CAD build for the part. Positions are in the model's coordinates, mm. Face numbers are marked on the shaded views. A direction names the side the tool comes from. Round coordinates to 2 decimals unless told otherwise and drop trailing zeros. Write each loop counter-clockwise with the first axis right and the second up, starting at its lowest first coordinate (ties: lowest second). Pieces come first, ordered by that corner, then holes. Notation, with made-up numbers: (30, 42) - (49, 42) arc R16 cw to (49, 66) - close; hole circle Ø9 at (69.5, -4.5). An arc over 180 degrees is marked (long way). Put each result on its own line as item: value. Start each with the question number.
Item 1: Mould opens along X. For the marked faces 4, 5 and 6 say: released by +X, released by -X, zero draft, split by the parting line, or undercut.
Item 2: Cut at B-B (x = 58). Give the cut face in (y, z), and give its area (3 significant figures).
Item 3: Pin check, flat tips, straight feed: pin 1 Ø2 at (x, z) = (11.5, 50.5) entering from -Y; pin 2 Ø12.5 at (y, z) = (-43, -43) entering from +X; pin 3 Ø5 at (y, z) = (51.5, 5.5) entering from +X; pin 4 Ø16 at (y, z) = (43, -43) entering from +X. Stop position of each tip, or through.
Item 4: Cut at A-A (z = 59.5). Give the cut face in (x, y).
Item 5: 3-axis set-ups, long thin cutter, end or side, ignore diameter. For the marked faces 1, 2 and 3: which of +Z, -Z, +X, -X, +Y, -Y reach the whole face in a straight line?
Item 6: Drill centre lines: line 1 (Y direction, x = 10.5, z = 43); line 2 (X direction, y = 36, z = -19); line 3 (Y direction, x = 58.5, z = 40). Where is each one in solid material? Low to high. Write a range as from..to.
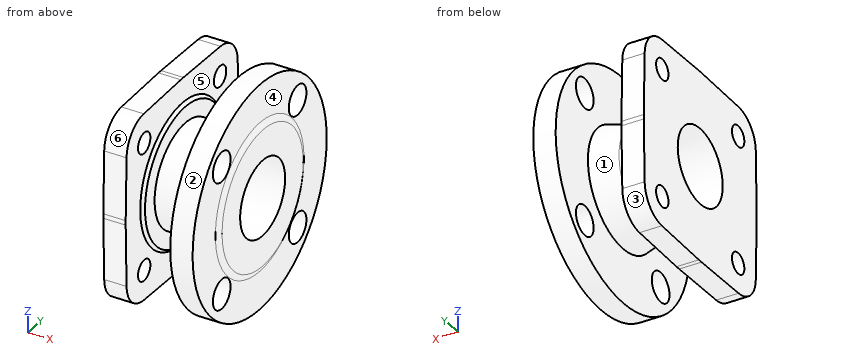
```python
from build123d import *

# Parameters (mm, degrees)
BOSS_EXTRUDE1_DEPTH = 15
SKETCH3_R           = 7
CUT_EXTRUDE1_DEPTH  = 15
SKETCH7_R           = 25.5
CUT_EXTRUDE2_DEPTH  = 128.72235513
SKETCH10_R          = 10
CUT_EXTRUDE3_DEPTH  = 25


with BuildPart() as part:
    # Sketch2 → Boss-Extrude1 (new body)
    with BuildSketch(Plane(origin=(0, 0, 0), x_dir=(0, 0, -1), z_dir=(1, 0, 0))):
        with BuildLine():
            Line((62.994461331, -43.470654948), (63.982276259, -1.506095834))
            ThreePointArc((63.982276259, -1.506095834), (64, 0), (63.982276259, 1.506095834))
            Line((63.982276259, 1.506095834), (62.994461331, 43.470654948))
            ThreePointArc((62.994461331, 43.470654948), (57.142135624, 57.142135624), (43.470654948, 62.994461331))
            Line((43.470654948, 62.994461331), (1.506095834, 63.982276259))
            ThreePointArc((1.506095834, 63.982276259), (0, 64), (-1.506095834, 63.982276259))
            Line((-1.506095834, 63.982276259), (-43.470654948, 62.994461331))
            ThreePointArc((-43.470654948, 62.994461331), (-57.142135624, 57.142135624), (-62.994461331, 43.470654948))
            Line((-62.994461331, 43.470654948), (-63.982276259, 1.506095834))
            ThreePointArc((-63.982276259, 1.506095834), (-64, 0), (-63.982276259, -1.506095834))
            Line((-63.982276259, -1.506095834), (-62.994461331, -43.470654948))
            ThreePointArc((-62.994461331, -43.470654948), (-57.142135624, -57.142135624), (-43.470654948, -62.994461331))
            Line((-43.470654948, -62.994461331), (-1.506095834, -63.982276259))
            ThreePointArc((-1.506095834, -63.982276259), (0, -64), (1.506095834, -63.982276259))
            Line((1.506095834, -63.982276259), (43.470654948, -62.994461331))
            ThreePointArc((43.470654948, -62.994461331), (57.142135624, -57.142135624), (62.994461331, -43.470654948))
        make_face()
    extrude(amount=BOSS_EXTRUDE1_DEPTH)

    # Sketch3 → Cut-Extrude1 (cut)
    with BuildSketch(Plane(origin=(15, 0, 0), x_dir=(0, 0, -1), z_dir=(1, 0, 0))):
        with Locations((-43, 43)):
            Circle(SKETCH3_R)
        with Locations(Location((43, 43, 0), (0, 0, 180))):
            Circle(SKETCH3_R)
        with Locations((43, -43)):
            Circle(SKETCH3_R)
        with Locations(Location((-43, -43, 0), (0, 0, 180))):
            Circle(SKETCH3_R)
    extrude(amount=-CUT_EXTRUDE1_DEPTH, mode=Mode.SUBTRACT)

    # Sketch4 → Revolve1 (revolve)
    with BuildSketch(Plane.XY, mode=Mode.PRIVATE) as revolve1_sk:
        Polygon((15, 0), (15, 47.5), (17, 45.5), (17, 34.6), (34, 34.6), (52, 39.423085464), (52, 76), (67, 76), (67, 50.228310139), (69, 46), (69, 0), align=None)
    revolve(revolve1_sk.sketch.rotate(Axis((69, 0, 0), (-1, 0, 0)), 90), axis=Axis((69, 0, 0), (-1, 0, 0)))

    # Sketch7 → Cut-Extrude2 (cut, through all)
    with BuildSketch(Plane(origin=(69, 0, 0), x_dir=(0, 0, -1), z_dir=(1, 0, 0))):
        Circle(SKETCH7_R)
    extrude(amount=-CUT_EXTRUDE2_DEPTH, mode=Mode.SUBTRACT)

    # Sketch10 → Cut-Extrude3 (cut)
    with BuildSketch(Plane(origin=(67, 0, 0), x_dir=(0, 0, -1), z_dir=(1, 0, 0))):
        with Locations((-43, 43)):
            Circle(SKETCH10_R)
        with Locations(Location((43, 43, 0), (0, 0, 180))):
            Circle(SKETCH10_R)
        with Locations((43, -43)):
            Circle(SKETCH10_R)
        with Locations(Location((-43, -43, 0), (0, 0, 180))):
            Circle(SKETCH10_R)
    extrude(amount=-CUT_EXTRUDE3_DEPTH, mode=Mode.SUBTRACT)


solid = part.part
```
Output values:
1. face 4: released by +X
1. face 5: undercut
1. face 6: zero draft
2. outline: circle Ø152 at (0, 0); hole circle Ø20 at (-43, -43); hole circle Ø20 at (-43, 43); hole circle Ø51 at (0, 0); hole circle Ø20 at (43, -43); hole circle Ø20 at (43, 43)
2. area: 14,800 mm2
3. pin 1: y = -61.91
3. pin 2: through
3. pin 3: x = 67.44
3. pin 4: x = 15
4. outline: (0, -54.3) - (15, -54.3) - (15, 54.3) - (0, 54.3) - close; (52, -47.28) - (67, -47.28) - (67, 47.28) - (52, 47.28) - close
5. face 1: none
5. face 2: +X
5. face 3: -Z, +X, -X, +Y
6. line 1: -63.01..-50, -36..36, 50..63.01
6. line 2: 0..17, 52..69
6. line 3: -64.62..-52.54, -33.46..33.46, 52.54..64.62
